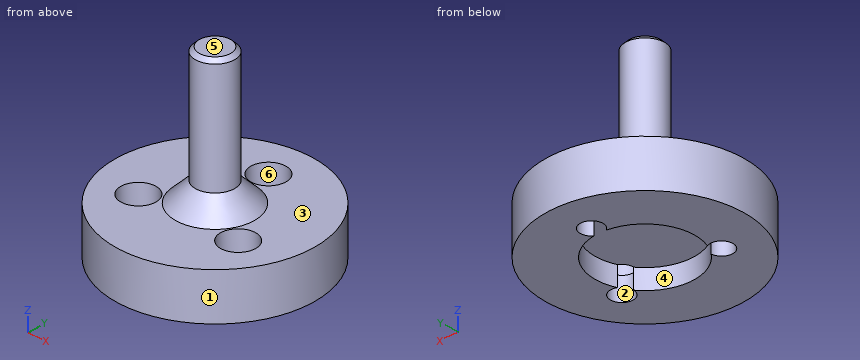
```python
from build123d import *

# Parameters (mm, degrees)
SKETCH1_R                    = 12.7
MOUNTING_FLANGE_DEPTH        = 6
SKETCH3_R                    = 6.35
MOTOR_SHAFT_RELIEF_DEPTH     = 2.54
SKETCH4_R                    = 1.45
SCREW_CLEARANCE_HOLES_DEPTH  = 19.936208702
SKETCH6_R                    = 2.25
SCREW_HEAD_COUNTERBORE_DEPTH = 3
SKETCH2_R                    = 2.5
BOSS_EXTRUDE1_DEPTH          = 17.272
CHAMFER1_SIZE                = 0.508
CHAMFER2_SIZE                = 2.54


with BuildPart() as part:
    # Sketch1 → Mounting Flange (new body)
    with BuildSketch(Plane.XY):
        Circle(SKETCH1_R)
    extrude(amount=MOUNTING_FLANGE_DEPTH)

    # Sketch3 → Motor Shaft Relief (cut)
    with BuildSketch(Plane(origin=(0, 0, 0), x_dir=(-1, 0, 0), z_dir=(0, 0, -1))):
        Circle(SKETCH3_R)
    extrude(amount=-MOTOR_SHAFT_RELIEF_DEPTH, mode=Mode.SUBTRACT)

    # Sketch4 → Screw Clearance Holes (cut, through all)
    with BuildSketch(Plane.XY.offset(6)):
        with Locations((0, 7.5)):
            Circle(SKETCH4_R)
        with Locations((6.495190528, -3.75)):
            Circle(SKETCH4_R)
        with Locations((-6.495190528, -3.75)):
            Circle(SKETCH4_R)
    extrude(amount=-SCREW_CLEARANCE_HOLES_DEPTH, mode=Mode.SUBTRACT)

    # Sketch6 → Screw Head Counterbore (cut)
    with BuildSketch(Plane.XY.offset(6)):
        with Locations((0, 7.5)):
            Circle(SKETCH6_R)
        with Locations((-6.495190528, -3.75)):
            Circle(SKETCH6_R)
        with Locations((6.495190528, -3.75)):
            Circle(SKETCH6_R)
    extrude(amount=-SCREW_HEAD_COUNTERBORE_DEPTH, mode=Mode.SUBTRACT)

    # Sketch2 → Boss-Extrude1 (add)
    with BuildSketch(Plane.XY.offset(6)):
        Circle(SKETCH2_R)
    extrude(amount=BOSS_EXTRUDE1_DEPTH)

    # Chamfer1
    chamfer1_edges = [part.edges().sort_by_distance(p)[0] for p in [
        (-2.5, 0, 23.272),
    ]]
    chamfer(chamfer1_edges, length=CHAMFER1_SIZE)

    # Chamfer2
    chamfer2_edges = [part.edges().sort_by_distance(p)[0] for p in [
        (-2.5, 0, 6),
    ]]
    chamfer(chamfer2_edges, length=CHAMFER2_SIZE)


solid = part.part
```
Geometry check sheet. Reference: the model listing, model coordinates, mm. Face numbers are marked on the shaded views. A direction names the side the tool comes from. Round coordinates to 2 decimals unless told otherwise and drop trailing zeros. Order: outer loops, then holes, each group sorted by start corner. A loop starts at its lowest first (then second) coordinate and runs counter-clockwise, first axis right, second up. Notation, with made-up numbers: (50.25, -21) - (80.25, -21) arc R13 ccw to (80.25, -7) - close; hole circle Ø9 at (36.25, 85.5). An arc over 180 degrees is marked (long way). Use a Markdown table: item, result. Add a question column.
(1) Sectioned sample at C-C, the plane z = 4. Enter the section's corners in (x, y).
(2) Tool access check on the marked faces 4, 5 and 6. Record the directions out of +Z, -Z, +X, -X, +Y, -Y that give a thin tool (end or side, any length) a straight path to the whole face; none if there is none.
(3) Sectioned sample at A-A, the plane x = 0. Enter the section's corners in (y, z), and give its area (3 significant figures).
(4) Release check for a two-part mould opening along Y. For the marked faces 1, 2 and 3 record: pulls with the +Y half, pulls with the -Y half, needs draft (parallel to the pull), parting line crosses it, or undercut.
(5) Depth check by flat-ended pin: pin 1 (3 mm diameter, centred on x = -8.5, z = 5, fed in from -Y); pin 2 (10 mm diameter, centred on y = 1, z = 21, fed in from -X); pin 3 (3.5 mm diameter, centred on x = -6.5, y = -3.75, fed in from -Z); pin 4 (1.3 mm diameter, centred on x = 7, y = -3, fed in from +Z). Enter the tip coordinate at first touch or a pass-through.
(6) Sectioned sample at B-B, the plane y = 0. Enter the section's corners in (x, z).
(7) Sectioned sample at D-D, the plane y = 7.5. Enter the section's corners in (x, z), and give its area (3 significant figures).
(8) Material ranges on line 1 along Y through (x, z) = (0, 4.8); line 2 along Y through (x, z) = (0, 2.15); line 3 along Z through (x, y) = (-1.5, -4.75), recorded low to high. Write a range as [from, to].
Answers below:
| question | item | result |
|---|---|---|
| 1 | outline | circle Ø25.4 at (0, 0); hole circle Ø4.5 at (-6.5, -3.75); hole circle Ø4.5 at (0, 7.5); hole circle Ø4.5 at (6.5, -3.75) |
| 2 | face 4 | -Z |
| 2 | face 5 | +Z, +X, -X, +Y, -Y |
| 2 | face 6 | +Z |
| 3 | outline | (-12.7, 0) - (-6.35, 0) - (-6.35, 2.54) - (6.05, 2.54) - (6.05, 3) - (5.25, 3) - (5.25, 6) - (5.04, 6) - (2.5, 8.54) - (2.5, 22.76) - (1.99, 23.27) - (-1.99, 23.27) - (-2.5, 22.76) - (-2.5, 8.54) - (-5.04, 6) - (-12.7, 6) - close; (8.95, 0) - (12.7, 0) - (12.7, 6) - (9.75, 6) - (9.75, 3) - (8.95, 3) - close |
| 3 | area | 191 mm² |
| 4 | face 1 | parting line crosses it |
| 4 | face 2 | undercut |
| 4 | face 3 | needs draft |
| 5 | pin 1 | y = -10.6 |
| 5 | pin 2 | x = -2.5 |
| 5 | pin 3 | z = 0 |
| 5 | pin 4 | z = 3 |
| 6 | outline | (-12.7, 0) - (-6.35, 0) - (-6.35, 2.54) - (6.35, 2.54) - (6.35, 0) - (12.7, 0) - (12.7, 6) - (5.04, 6) - (2.5, 8.54) - (2.5, 22.76) - (1.99, 23.27) - (-1.99, 23.27) - (-2.5, 22.76) - (-2.5, 8.54) - (-5.04, 6) - (-12.7, 6) - close |
| 7 | outline | (-10.25, 0) - (-1.45, 0) - (-1.45, 3) - (-2.25, 3) - (-2.25, 6) - (-10.25, 6) - close; (1.45, 0) - (10.25, 0) - (10.25, 6) - (2.25, 6) - (2.25, 3) - (1.45, 3) - close |
| 7 | area | 101 mm² |
| 8 | line 1 | [-12.7, 5.25], [9.75, 12.7] |
| 8 | line 2 | [-12.7, -6.35], [8.95, 12.7] |
| 8 | line 3 | [2.54, 6.06] |
